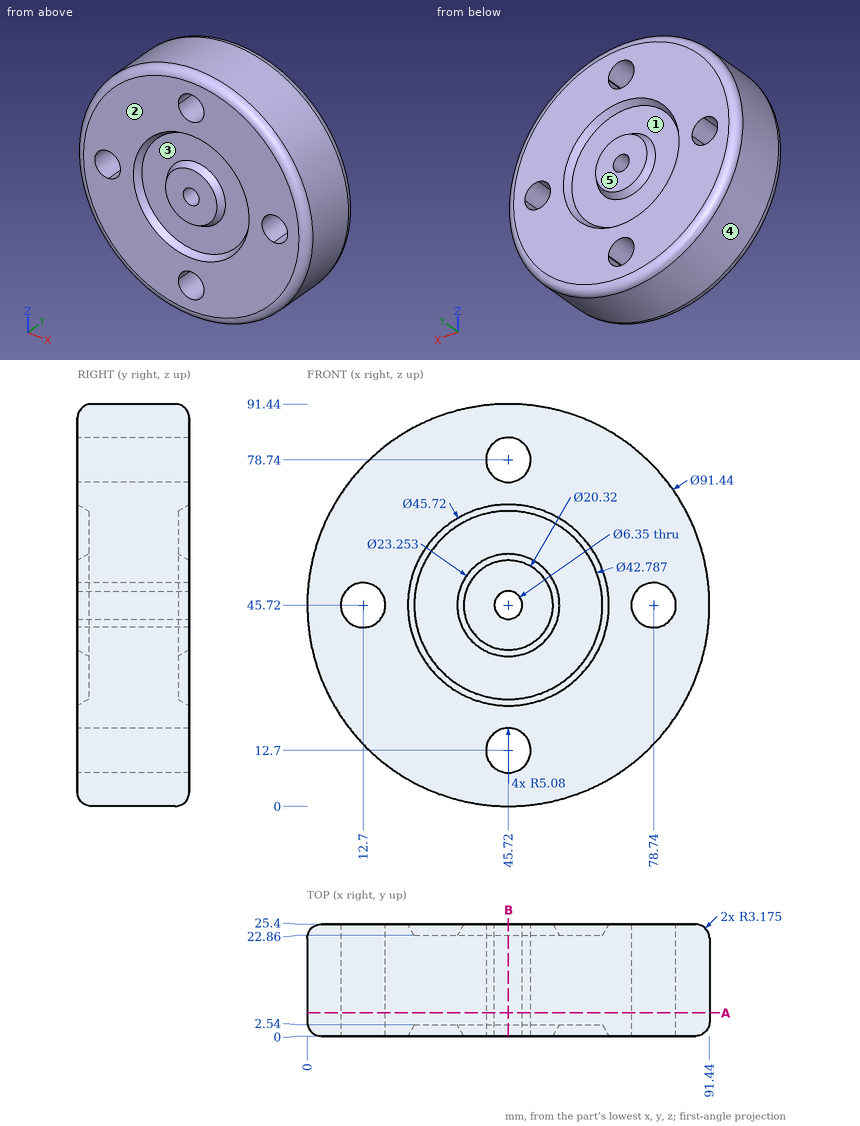
Source: three-view drawing plus pictorial views. Frame: mm from the lowest corner of the part. A direction names the side the tool comes from. Coordinates: 2 decimals unless noted, no trailing zeros. Order: outer loops, then holes, each group sorted by start corner. A loop starts at its lowest first (then second) coordinate and runs counter-clockwise, first axis right, second up.
Item 1: Pull-direction query (Z, two-part tool) for the marked faces 3, 4 and 5; classes: pulls with the +Z half, pulls with the -Z half, needs draft (parallel to the pull), parting line crosses it, or undercut.
Output values:
face 3: undercut
face 4: parting line crosses it
face 5: needs draft
Item 2: First-contact query: P1, Ø3, axis at x = 37, z = 28, coming from the +Y side; P2, Ø3, axis at x = 32.5, y = 5.5, coming from the +Z side; P3, Ø3, axis at x = 72, y = 5.5, coming from the +Z side. Flat tips, straight axial feed; report the tip coordinate or a pass-through.
Output values:
P1: stops at y = 22.86
P2: stops at z = 89.91
P3: stops at z = 84.14
Item 3: Set-up query: the marked faces 1 and 2. Return all of +Z, -Z, +X, -X, +Y, -Y with unobstructed straight access to the full face (end or side cutting, diameter ignored); none if empty.
Output values:
face 1: +Y
face 2: +Z, -Z, +X, -X, -Y
Item 4: Cut plane A-A (y = 5.25). Return loops of the section in (x, z) (3 decimals).
Output values:
outline: circle Ø91.44 at (45.72, 45.72); hole circle Ø10.16 at (12.7, 45.72); hole circle Ø10.16 at (45.72, 12.7); hole circle Ø10.16 at (45.72, 78.74); hole circle Ø6.35 at (45.72, 45.72); hole circle Ø10.16 at (78.74, 45.72)
Item 5: Material intervals for line 1 (Z direction, x = 47, y = 8.25); line 2 (X direction, y = 6.75, z = 50); line 3 (Z direction, x = 14, y = 15.5), sorted ascending.
Output values:
line 1: z = 0.02 to 7.78, 17.62 to 42.81, 48.63 to 73.82, 83.66 to 91.42
line 2: x = 0.2 to 9.96, 15.44 to 76, 81.48 to 91.24
line 3: z = 12.79 to 40.81, 50.63 to 78.65
Item 6: Cut plane B-B (x = 45.72). Count the separate pieces of the cut face and the enclosed holes in it, plus the area to 3 significant figures.
Output values:
separate pieces: 4
enclosed holes: 0
area: 1,520 mm2
